Source: CAD feature listing. Evaluate the final solid. Frame: model axes, mm. A direction names the side the tool comes from. Give positions to 0.01 mm unless a question says otherwise; leave off trailing zeros. Order: outer loops, then holes, each group sorted by start corner. A loop starts at its lowest first (then second) coordinate and runs counter-clockwise, first axis right, second up.
from build123d import *

# Parameters (mm, degrees)
SKETCH1_W           = 4
SKETCH1_H           = 2
BOSS_EXTRUDE1_DEPTH = 4
BOSS_EXTRUDE2_DEPTH = 2
SKETCH3_R           = 1
CUT_EXTRUDE1_DEPTH  = 3
BOSS_EXTRUDE4_DEPTH = 2
CUT_EXTRUDE2_DEPTH  = 1
SKETCH8_W           = 1
SKETCH8_H           = 2
BOSS_EXTRUDE5_DEPTH = 2
CUT_EXTRUDE3_DEPTH  = 1
BOSS_EXTRUDE6_DEPTH = 1
BOSS_EXTRUDE7_DEPTH = 1
BOSS_EXTRUDE8_DEPTH = 1


with BuildPart() as part:
    # Sketch1 → Boss-Extrude1 (new body)
    with BuildSketch(Plane.XY):
        Rectangle(SKETCH1_W, SKETCH1_H)
    extrude(amount=BOSS_EXTRUDE1_DEPTH)

    # Sketch2 → Boss-Extrude2 (add)
    with BuildSketch(Plane(origin=(0, 1, 0), x_dir=(1, 0, 0), z_dir=(0, 1, 0))):
        with BuildLine():
            Line((2, 0), (2, -4))
            ThreePointArc((2, -4), (4, -2), (2, 0))
        make_face()
    extrude(amount=-BOSS_EXTRUDE2_DEPTH)

    # Sketch3 → Cut-Extrude1 (cut, through all)
    with BuildSketch(Plane(origin=(0, 1, 0), x_dir=(1, 0, 0), z_dir=(0, 1, 0))):
        with Locations((2, -2)):
            Circle(SKETCH3_R)
    extrude(amount=-CUT_EXTRUDE1_DEPTH, mode=Mode.SUBTRACT)

    # Sketch4 → Boss-Extrude4 (add)
    with BuildSketch(Plane.ZY.offset(2)):
        with BuildLine():
            Line((0, 1), (0, 2))
            ThreePointArc((0, 2), (1.5, 3.5), (3, 2))
            Line((3, 2), (3, 1))
            Line((3, 1), (2, 1))
            Line((2, 1), (2, 2))
            ThreePointArc((2, 2), (1.5, 2.5), (1, 2))
            Line((1, 2), (1, 1))
            Line((1, 1), (0, 1))
        make_face()
    extrude(amount=-BOSS_EXTRUDE4_DEPTH)

    # Sketch7 → Cut-Extrude2 (cut)
    with BuildSketch(Plane(origin=(0, 0, 0), x_dir=(0, 0, -1), z_dir=(1, 0, 0))):
        with BuildLine():
            Line((-1.5, 2.5), (-1.5, 3.5))
            ThreePointArc((-1.5, 3.5), (-2.560660172, 3.060660172), (-3, 2))
            Line((-3, 2), (-2, 2))
            ThreePointArc((-2, 2), (-1.853553391, 2.353553391), (-1.5, 2.5))
        make_face()
    extrude(amount=-CUT_EXTRUDE2_DEPTH, mode=Mode.SUBTRACT)

    # Sketch8 → Boss-Extrude5 (add)
    with BuildSketch(Plane.ZY.offset(2)):
        with Locations((4.5, 0)):
            Rectangle(SKETCH8_W, SKETCH8_H)
    extrude(amount=-BOSS_EXTRUDE5_DEPTH)

    # Sketch9 → Cut-Extrude3 (cut)
    with BuildSketch(Plane.ZY.offset(2)):
        Polygon((5, 1), (4, 1), (5, -1), align=None)
    extrude(amount=-CUT_EXTRUDE3_DEPTH, mode=Mode.SUBTRACT)

    # Sketch10 → Boss-Extrude6 (add)
    with BuildSketch(Plane(origin=(0, -1, 0), x_dir=(-1, 0, 0), z_dir=(0, -1, 0))):
        with BuildLine():
            Line((0, -5), (-1, -5))
            Line((-1, -5), (-3.069693846, -3.689897949))
            ThreePointArc((-3.069693846, -3.689897949), (-2.556868074, -3.920910708), (-2, -4))
            Line((-2, -4), (0, -4))
            Line((0, -4), (0, -5))
        make_face()
    extrude(amount=-BOSS_EXTRUDE6_DEPTH)

    # Sketch11 → Boss-Extrude7 (add)
    with BuildSketch(Plane(origin=(0, 1, 0), x_dir=(1, 0, 0), z_dir=(0, 1, 0))):
        Polygon((0, -3), (0, -5), (-1, -5), (-1, -4), (-2, -4), (-2, -3), align=None)
    extrude(amount=BOSS_EXTRUDE7_DEPTH)

    # Sketch12 → Boss-Extrude8 (add)
    with BuildSketch(Plane.ZY.offset(1)):
        Polygon((4, 2), (5, -1), (4, 1), align=None)
    extrude(amount=BOSS_EXTRUDE8_DEPTH)


solid = part.part
(1) Line query: line 1 along Z through (x, y) = (2, 0.4); line 2 along Y through (x, z) = (-1.25, 3.5); line 3 along X through (y, z) = (-0.4, 2). Output: solid intervals per line, ascending.
(2) Section D-D, the plane z = 2.5. Return loops of the section in (x, y).
(3) Pin query (flat end, axial travel): pin 1 Ø0.6 at (y, z) = (1.5, 3) entering from +X; pin 2 Ø3 at (x, z) = (2, 2) entering from +Y; pin 3 Ø1.6 at (x, z) = (-0.5, 3) entering from +Y. Return the tip coordinate at first contact, or that it passes through.
(4) Section B-B, the plane x = -1.15. Return loops of the section in (y, z).
(5) Section A-A, the plane y = 1.4. Return loops of the section in (x, z), plus the area to 3 significant figures.
(6) Access query for faces 5 (the flat face through (-0.8, 2, 3.5)), 6 (the cylindrical face through (4, 0, 2)), 7 (the flat face through (1, 1, 1)). Directions: +Z, -Z, +X, -X, +Y, -Y. A direction counts if a zero-diameter tool reaches every point of the face in a straight line with its end or side. Return the directions, or none.
(7) Section C-C, the plane x = 0.6. Return loops of the section in (y, z).
(8) Draft query along Y for faces 1 (the flat face through (-1, 3, 2)), 2 (the flat face through (0, -1, 2)), 3 (the flat face through (-1, 1.5, 1)), 4 (the cylindrical face through (-1.24, 3.4, 0.96)). Return one class per face: +Y half, -Y half, draft (parallel to the pull), parting line (faces both ways), or undercut.
Checks:
1. line 1: z = 0 to 1, 3 to 4
1. line 2: y = -1 to 2
1. line 3: x = -2 to 1, 3 to 4
2. outline: (-2, -1) - (1.13, -1) - (1.13, 1) - (0, 1) - (0, 2) - (-1, 2) - (-1, 3.12) - (-2, 3.12) - close; (2.87, -1) - (3.94, -1) - (3.94, 1) - (2.87, 1) - close
3. pin 1: stops at x = 0
3. pin 2: stops at y = 1
3. pin 3: stops at y = 3.22
4. outline: (-1, 0) - (2, 0) arc R1.5 ccw to (2, 3) - (2, 4) - (-1, 5) - close; hole (1, 1) - (2, 1) arc R0.5 ccw to (2, 2) - (1, 2) - close
5. outline: (-2, 0) - (0, 0) - (0, 1) - (-2, 1) - close; (-2, 2) - (0, 2) - (0, 5) - (-1, 5) - (-1, 4.2) - (-2, 4.2) - close
5. area: 7.20 mm2
6. face 5: +Z, +X, +Y
6. face 6: +X, +Y
6. face 7: +X
7. outline: (-1, 0) - (1, 0) - (1, 4) - (0, 4) - (0, 5) - (-1, 5) - close
8. face 1: draft
8. face 2: -Y half
8. face 3: undercut
8. face 4: +Y half
